Source: CAD feature listing. Evaluate the final solid. Frame: model axes, mm. Face numbers are marked on the shaded views. A direction names the side the tool comes from. Give positions to 0.01 mm unless a question says otherwise; leave off trailing zeros. Write each loop counter-clockwise with the first axis right and the second up, starting at its lowest first coordinate (ties: lowest second). Pieces come first, ordered by that corner, then holes. Notation, with made-up numbers: M 78,-6.75 L 137,-6.75 A25 ccw 137,14.25 Z; hole C -14.75,78.25 d10. An arc over 180 degrees is marked long. Answer as a JSON object with one key per item and string values. Group by question number.
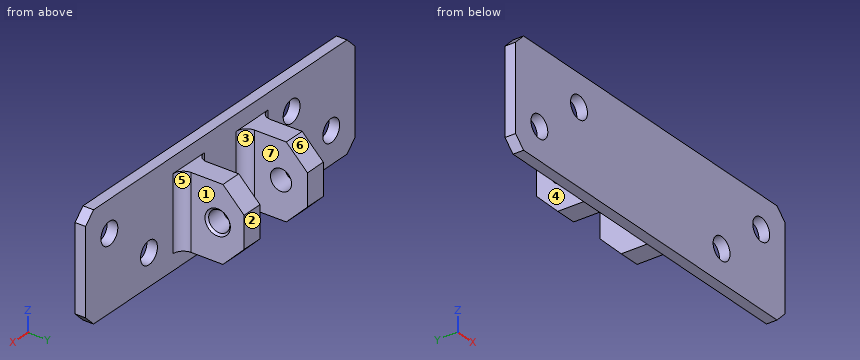
```python
from build123d import *

# Parameters (mm, degrees)
SKETCH1_W               = 107.95
SKETCH1_H               = 31.75
BOSS_EXTRUDE1_DEPTH     = 1.5875
F_1_4_CLEARANCE_HOLE1_D = 6.7564
SKETCH4_W               = 6.35
SKETCH4_H               = 22.225
BOSS_EXTRUDE2_DEPTH     = 19.05
CHAMFER2_SIZE           = 3.175
FILLET1_R               = 3.175
CHAMFER3_SIZE           = 6.35


with BuildPart() as part:
    # Sketch1 → Boss-Extrude1 (new, symmetric)
    with BuildSketch(Plane(origin=(0, 0, 0), x_dir=(1, 0, 0), z_dir=(0, 1, 0))):
        Rectangle(SKETCH1_W, SKETCH1_H)
    extrude(amount=BOSS_EXTRUDE1_DEPTH, both=True)

    # 1/4 Clearance Hole1 (through all)
    with Locations(Plane(origin=(0, 1.5875, 0), x_dir=(1, 0, 0), z_dir=(0, 1, 0))):
        with Locations((-44.45, 6.35), (28.575, 6.35), (-28.575, -6.35), (44.45, -6.35)):
            Hole(F_1_4_CLEARANCE_HOLE1_D / 2)

    # Sketch4 → Boss-Extrude2 (add)
    with BuildSketch(Plane(origin=(0, 1.5875, 0), x_dir=(1, 0, 0), z_dir=(0, 1, 0))):
        with Locations((-12.7, 0)):
            Rectangle(SKETCH4_W, SKETCH4_H)
        with Locations((12.7, 0)):
            Rectangle(SKETCH4_W, SKETCH4_H)
    extrude(amount=BOSS_EXTRUDE2_DEPTH)

    # Chamfer2
    chamfer2_edges = [part.edges().sort_by_distance(p)[0] for p in [
        (-53.975, 0, -15.875),
        (53.975, 0, -15.875),
        (53.975, 0, 15.875),
        (-53.975, 0, 15.875),
    ]]
    chamfer(chamfer2_edges, length=CHAMFER2_SIZE)

    # Fillet1
    fillet1_edges = [part.edges().sort_by_distance(p)[0] for p in [
        (-15.875, 1.5875, 0),
        (-9.525, 1.5875, 0),
        (9.525, 1.5875, 0),
        (15.875, 1.5875, 0),
    ]]
    fillet(fillet1_edges, radius=FILLET1_R)

    # Sketch6 → 1/4 (0.25) Diameter Hole1 (revolve, cut)
    with BuildSketch(Plane(origin=(15.875, 12.7, 0), x_dir=(0, 0, -1), z_dir=(0, 1, 0))):
        Polygon((0, 0), (0, 31.75), (3.81, 31.75), (3.175, 31.115), (3.175, 0.635), (3.81, 0), align=None)
    revolve(axis=Axis((22.225, 12.7, 0), (-1, 0, 0)), mode=Mode.SUBTRACT)

    # Chamfer3
    chamfer3_edges = [part.edges().sort_by_distance(p)[0] for p in [
        (-12.7, 20.6375, 11.1125),
        (-12.7, 20.6375, -11.1125),
        (12.7, 20.6375, 11.1125),
        (12.7, 20.6375, -11.1125),
    ]]
    chamfer(chamfer3_edges, length=CHAMFER3_SIZE)


solid = part.part
```
(1) Section C-C, the plane x = 44.45. Return loops of the section in (y, z) (1 decimal).
(2) Section D-D, the plane y = 6. Return loops of the section in (x, z) (1 decimal).
(3) Ray query, L1, parallel to X at y = 17, z = -7.5 (3 decimals); L2, parallel to Z at x = 44.45, y = -0.9 (3 decimals); L3, parallel to X at y = 1.5, z = -6.5 (3 decimals). Return the intervals inside material, ascending. Write a range as [from, to].
(4) Pull-direction query (X, two-part tool) for the marked faces 4, 5, 6 and 7; classes: pulls with the +X half, pulls with the -X half, needs draft (parallel to the pull), parting line crosses it, or undercut.
(5) Section A-A, the plane z = -6.35. State how many separate pieces and enclosed holes the cut face has, plus the area to 3 significant figures.
(6) Contact query for flat-ended pins moving along their axis: pin 1 Ø12.5 at (y, z) = (10, 1) entering from -X; pin 2 Ø5.5 at (x, z) = (-44.45, -6.35) entering from -Y; pin 3 Ø4 at (x, y) = (-14.5, 10.5) entering from -Z; pin 4 Ø4 at (x, y) = (11, 9) entering from +Z. Output: stop coordinate, or through.
(7) Section B-B, the plane y = 12.7. Return loops of the section in (x, z) (1 decimal).
(8) Access query for the marked faces 1, 2 and 3. Directions: +Z, -Z, +X, -X, +Y, -Y. A direction counts if a zero-diameter tool reaches every point of the face in a straight line with its end or side. Return the directions, or none.
Reported:
{
 "1": {"outline": "M -1.6,-15.9 L 1.6,-15.9 L 1.6,3 L -1.6,3 Z; M -1.6,9.7 L 1.6,9.7 L 1.6,15.9 L -1.6,15.9 Z"},
 "2": {"outline": "M -15.9,-11.1 L -9.5,-11.1 L -9.5,11.1 L -15.9,11.1 Z; M 9.5,-11.1 L 15.9,-11.1 L 15.9,11.1 L 9.5,11.1 Z"},
 "3": {"L1": "x = [-15.875, -9.525], [9.525, 15.875]", "L2": "z = [-15.875, 2.972], [9.728, 15.875]", "L3": "x = [-53.975, -47.825], [-41.075, 25.2], [31.95, 53.975]"},
 "4": {"face 4": "pulls with the -X half", "face 5": "pulls with the +X half", "face 6": "needs draft", "face 7": "undercut"},
 "5": {"separate pieces": "3", "enclosed holes": "0", "area": "530 mm2"},
 "6": {"pin 1": "stops at x = -16.04", "pin 2": "passes through", "pin 3": "stops at z = -11.11", "pin 4": "stops at z = 11.11"},
 "7": {"outline": "M -15.9,-11.1 L -9.5,-11.1 L -9.5,-3.2 L -15.2,-3.2 L -15.9,-3.8 Z; M -15.9,3.8 L -15.2,3.2 L -9.5,3.2 L -9.5,11.1 L -15.9,11.1 Z; M 9.5,-11.1 L 15.9,-11.1 L 15.9,-3.8 L 15.2,-3.2 L 9.5,-3.2 Z; M 9.5,3.2 L 15.2,3.2 L 15.9,3.8 L 15.9,11.1 L 9.5,11.1 Z"},
 "8": {"face 1": "+Z, -Z, +X, +Y", "face 2": "+Z, -Z, +X, -X, +Y", "face 3": "+Z, -Z, +Y"}
}
